from build123d import *

# Parameters (mm, degrees)
SKETCH2_W                                          = 40
SKETCH2_H                                          = 12
BOSS_EXTRUDE1_DEPTH                                = 24
CBORE_FOR_M2_5_HEX_HEAD_MACHINE_SCREW1_D           = 3
CBORE_FOR_M2_5_HEX_HEAD_MACHINE_SCREW1_DEPTH       = 38.1
CBORE_FOR_M2_5_HEX_HEAD_MACHINE_SCREW1_CBORE_D     = 6
CBORE_FOR_M2_5_HEX_HEAD_MACHINE_SCREW1_CBORE_DEPTH = 4
CBORE_FOR_M2_5_HEX_HEAD_MACHINE_SCREW1_TIP         = 0.901290929
SKETCH11_W                                         = 40
SKETCH11_H                                         = 5.5
BOSS_EXTRUDE2_DEPTH                                = 10
SKETCH12_W                                         = 40
SKETCH12_H                                         = 7.5
BOSS_EXTRUDE3_DEPTH                                = 18.5
SKETCH10_R                                         = 4.05
CUT_EXTRUDE1_DEPTH                                 = 17
CUT_EXTRUDE1_DEPTH_BACK                            = 6
SKETCH13_R                                         = 4.8
CUT_EXTRUDE2_DEPTH                                 = 5.5
SKETCH14_R                                         = 10.05
CUT_EXTRUDE3_DEPTH                                 = 2.1
TAP_DRILL_FOR_M2_5_HELICOIL1_D                     = 2.65
FILLET1_R                                          = 11
FILLET2_R                                          = 9


with BuildPart() as part:
    # Sketch2 → Boss-Extrude1 (new body)
    with BuildSketch(Plane(origin=(0, 0, 0), x_dir=(1, 0, 0), z_dir=(0, 1, 0))):
        with Locations((20, 6)):
            Rectangle(SKETCH2_W, SKETCH2_H)
    extrude(amount=BOSS_EXTRUDE1_DEPTH)

    # CBORE for M2.5 Hex Head Machine Screw1
    with Locations(Plane(origin=(0, 24, 0), x_dir=(1, 0, 0), z_dir=(0, 1, 0))):
        with Locations((7.5, 6.5), (32.5, 6.5)):
            CounterBoreHole(CBORE_FOR_M2_5_HEX_HEAD_MACHINE_SCREW1_D / 2, CBORE_FOR_M2_5_HEX_HEAD_MACHINE_SCREW1_CBORE_D / 2, CBORE_FOR_M2_5_HEX_HEAD_MACHINE_SCREW1_CBORE_DEPTH, depth=CBORE_FOR_M2_5_HEX_HEAD_MACHINE_SCREW1_DEPTH)
            with Locations((0, 0, -(CBORE_FOR_M2_5_HEX_HEAD_MACHINE_SCREW1_DEPTH + CBORE_FOR_M2_5_HEX_HEAD_MACHINE_SCREW1_TIP / 2))):  # 118° drill point
                Cone(0, CBORE_FOR_M2_5_HEX_HEAD_MACHINE_SCREW1_D / 2, CBORE_FOR_M2_5_HEX_HEAD_MACHINE_SCREW1_TIP, mode=Mode.SUBTRACT)

    # Sketch11 → Boss-Extrude2 (add)
    with BuildSketch(Plane(origin=(0, 0, -12), x_dir=(-1, 0, 0), z_dir=(0, 0, -1))):
        with Locations((-20, 2.75)):
            Rectangle(SKETCH11_W, SKETCH11_H)
    extrude(amount=BOSS_EXTRUDE2_DEPTH)

    # Sketch12 → Boss-Extrude3 (add)
    with BuildSketch(Plane(origin=(0, 5.5, 0), x_dir=(1, 0, 0), z_dir=(0, 1, 0))):
        with Locations((20, 18.25)):
            Rectangle(SKETCH12_W, SKETCH12_H)
    extrude(amount=BOSS_EXTRUDE3_DEPTH)

    # Sketch10 → Cut-Extrude1 (cut, two sides)
    with BuildSketch(Plane(origin=(0, 0, -12), x_dir=(-1, 0, 0), z_dir=(0, 0, -1))) as cut_extrude1_sk:
        with Locations((-20, 17.7)):
            Circle(SKETCH10_R)
    extrude(amount=CUT_EXTRUDE1_DEPTH, mode=Mode.SUBTRACT)
    extrude(cut_extrude1_sk.sketch, amount=-CUT_EXTRUDE1_DEPTH_BACK, mode=Mode.SUBTRACT)

    # Sketch13 → Cut-Extrude2 (cut)
    with BuildSketch(Plane(origin=(0, 0, -22), x_dir=(-1, 0, 0), z_dir=(0, 0, -1))):
        with Locations((-20, 17.7)):
            Circle(SKETCH13_R)
    extrude(amount=-CUT_EXTRUDE2_DEPTH, mode=Mode.SUBTRACT)

    # Sketch14 → Cut-Extrude3 (cut)
    with BuildSketch(Plane(origin=(0, 0, -22), x_dir=(-1, 0, 0), z_dir=(0, 0, -1))):
        with Locations((-20, 17.7)):
            Circle(SKETCH14_R)
    extrude(amount=-CUT_EXTRUDE3_DEPTH, mode=Mode.SUBTRACT)

    # Tap Drill for M2.5 Helicoil1 (through all)
    with Locations(Plane(origin=(0, 0, -6), x_dir=(-1, 0, 0), z_dir=(0, 0, -1))):
        with Locations((-20, 17.7)):
            Hole(TAP_DRILL_FOR_M2_5_HELICOIL1_D / 2)

    # Fillet1
    fillet1_edges = [part.edges().sort_by_distance(p)[0] for p in [
        (40, 12, 0),
        (0, 12, 0),
    ]]
    fillet(fillet1_edges, radius=FILLET1_R)

    # Fillet2
    fillet2_edges = [part.edges().sort_by_distance(p)[0] for p in [
        (0, 12, -22),
        (40, 12, -22),
    ]]
    fillet(fillet2_edges, radius=FILLET2_R)


solid = part.part
Could you check a few things on this model? Use its own coordinates, in mm. A direction names the side the tool comes from. Give positions to 0.01 mm unless a question says otherwise; leave off trailing zeros. Loops run counter-clockwise (first coordinate to the right, second up) from the corner with the lowest first, then second, coordinate; pieces in that order, holes last. Notation, with made-up numbers: (-37.75, 74) -> (8.25, 74) arc R22 cw to (8.25, 90) -> close; hole circle Ø4 at (-13, 40). An arc over 180 degrees is marked (long way). Answer as CSV lines item,"result". Start each with the question number.
(1) I need wall thicknesses on probe 1 along X at (y, z) = (16, -6.5); probe 2 along Z at (x, y) = (14, 12); probe 3 along Z at (x, y) = (32.5, 11.5). Which ranges of each line are inside material? Lowest first, please.
(2) We'd pull the mould along Z, two halves only. Please class faces 4 (the cylindrical face through (29.5, 22, -6.6)), 5 (the cylindrical face through (8.7, 9.9, -5.6)), 6 (the flat face through (0, 9.2, -11.8)), 7 (the flat face through (20, 6, -22)): released by +Z, released by -Z, zero draft, split by the parting line, or undercut.
(3) If we section it at A-A on y = 6.5: Write out the boundary of the cut face in (x, z).
(4) If we section it at D-D on x = 20: Write out the boundary of the cut face in (y, z) (3 decimals).
(5) Which directions (+Z, -Z, +X, -X, +Y, -Y) give clear straight access to the entire face, cutting with the end or side of a thin tool? Please do faces 1 (the cylindrical face through (10.27, 22.03, -5.35)), 2 (the flat face through (22, 14, -16.5)), 3 (the flat face through (20, 13, -14.5)).
(6) If we section it at B-B on y = 17.7: Count the separate pieces of the cut face and the enclosed holes in it, then the cut area to 3 significant figures.
(7) If we section it at C-C on z = -6.5: Write out the boundary of the cut face in (x, y).
(8) I'm going to push flat-ended pins straight in: pin 1 Ø2.5 at (x, z) = (7.5, -6.5) entering from +Y; pin 2 Ø9 at (x, y) = (19, 19.5) entering from -Z; pin 3 Ø12 at (y, z) = (21.5, -3) entering from -X; pin 4 Ø3 at (x, y) = (20, 19) entering from -Z. Where does each tip first touch, or does it pass through?
Computed:
1,probe 1,"x = 0.96 to 6, 9 to 16.32, 23.68 to 31, 34 to 39.04"
1,probe 2,"z = -19.9 to -14.5, -12 to 0"
1,probe 3,"z = -21.87 to -14.5, -12 to -8, -5 to -0.57"
2,face 4,"undercut"
2,face 5,"undercut"
2,face 6,"zero draft"
2,face 7,"released by -Z"
3,outline,"(0, -12) -> (40, -12) -> (40, -11) arc R11 ccw to (29, 0) -> (11, 0) arc R11 ccw to (0, -11) -> close; (0.13, -14.5) arc R9 ccw to (9, -22) -> (31, -22) arc R9 ccw to (39.87, -14.5) -> close; hole circle Ø3 at (7.5, -6.5); hole circle Ø3 at (32.5, -6.5)"
4,outline,"(0, -22) -> (7.65, -22) -> (7.65, -19.9) -> (12.9, -19.9) -> (12.9, -16.5) -> (13.65, -16.5) -> (13.65, -14.5) -> (5.5, -14.5) -> (5.5, -12) -> (13.65, -12) -> (13.65, -6) -> (16.375, -6) -> (16.375, 0) -> (0, 0) -> close; (19.025, -6) -> (21.75, -6) -> (21.75, -12) -> (24, -12) -> (24, 0) -> (19.025, 0) -> close; (21.75, -16.5) -> (22.5, -16.5) -> (22.5, -19.9) -> (24, -19.9) -> (24, -14.5) -> (21.75, -14.5) -> close"
5,face 1,"+Y"
5,face 2,"-Z"
5,face 3,"+X, -X, +Y"
6,separate pieces,"4"
6,enclosed holes,"2"
6,area,"524 mm2"
7,outline,"(0.96, 0) -> (6, 0) -> (6, 20) -> (4.5, 20) -> (4.5, 24) -> (0.96, 24) -> close; (9, 0) -> (31, 0) -> (31, 20) -> (29.5, 20) -> (29.5, 24) -> (10.5, 24) -> (10.5, 20) -> (9, 20) -> close; (34, 0) -> (39.04, 0) -> (39.04, 24) -> (35.5, 24) -> (35.5, 20) -> (34, 20) -> close; hole circle Ø8.1 at (20, 17.7)"
8,pin 1,"passes through"
8,pin 2,"stops at z = -19.9"
8,pin 3,"stops at x = 0.18"
8,pin 4,"stops at z = -6"
